Verification items for the finished model (mm, model axes). A direction names the side the tool comes from. Round coordinates to 2 decimals unless told otherwise and drop trailing zeros. Loops run counter-clockwise (first coordinate to the right, second up) from the corner with the lowest first, then second, coordinate; pieces in that order, holes last. Notation, with made-up numbers: M 68.25,52.25 L 99.25,52.25 A36 ccw 99.25,91.25 Z; hole C 79.5,11.5 d1. An arc over 180 degrees is marked long. Answer as CSV lines item,"result".
```python
from build123d import *

# Parameters (mm, degrees)
F0_W     = 61.967217
F0_H     = 89.508198
F1_DEPTH = 7.5
F2_T     = -1.5


with BuildPart() as f1:
    # F0 (on Front) → F1 (new body, symmetric)
    with BuildSketch(Plane.XZ):
        with Locations((2.868853, 12.47951)):
            Rectangle(F0_W, F0_H)
    extrude(amount=F1_DEPTH, both=True)

    # F2
    f2_openings = [f1.faces().sort_by_distance(p)[0] for p in [
        (2.868854, -7.5, 12.47951),
    ]]
    offset(amount=F2_T, openings=f2_openings)


solid = f1.part
```
1) Go/stop test with a flat-tipped pin: pin 1 (8 mm diameter, centred on x = 14.5, z = -16, fed in from -Y). Record where the tip stops, or that it passes through.
Here are the results:
pin 1,"stops at y = 6"
2) Section check C-C (z = 32.5). Record the cut outline in (x, y).
Here are the results:
outline,"M -28.11,-7.5 L -26.61,-7.5 L -26.61,6 L 32.35,6 L 32.35,-7.5 L 33.85,-7.5 L 33.85,7.5 L -28.11,7.5 Z"
3) Section check B-B (x = -9). Record the cut outline in (y, z), plus the area to 3 significant figures.
Here are the results:
outline,"M -7.5,-32.27 L 7.5,-32.27 L 7.5,57.23 L -7.5,57.23 L -7.5,55.73 L 6,55.73 L 6,-30.77 L -7.5,-30.77 Z"
area,"175 mm^2"
4) Section check A-A (y = -5.75). Record the cut outline in (x, z), plus the area to 3 significant figures.
Here are the results:
outline,"M -28.11,-32.27 L 33.85,-32.27 L 33.85,57.23 L -28.11,57.23 Z; hole M -26.61,-30.77 L 32.35,-30.77 L 32.35,55.73 L -26.61,55.73 Z"
area,"445 mm^2"
5) Material ranges on probe 1 along X at (y, z) = (-5.25, 24); probe 2 along Z at (x, y) = (-9, -0.5); probe 3 along Y at (x, z) = (17.5, 37.5), recorded low to high.
Here are the results:
probe 1,"x = -28.11 to -26.61, 32.35 to 33.85"
probe 2,"z = -32.27 to -30.77, 55.73 to 57.23"
probe 3,"y = 6 to 7.5"
6) Set-up check for faces 1 (the flat face through (2, -1, 55.734)), 2 (the flat face through (2, 0, 57.234)): record each of +Z, -Z, +X, -X, +Y, -Y from which the full face is reachable in a straight line by a thin tool's end or side.
Here are the results:
face 1,"-Y"
face 2,"+Z, +X, -X, +Y, -Y"
7) Draft check along X on faces 3 (the flat face through (3, -7.5, 56)), 4 (the flat face through (-28.115, 0, 12)), 5 (the flat face through (32.352, -1, 12)). Enter one of: +X half, -X half, draft (parallel to the pull), parting line (faces both ways), or undercut.
Here are the results:
face 3,"draft"
face 4,"-X half"
face 5,"undercut"
